from build123d import *

# Parameters (mm, degrees)
F1_DEPTH  = 16
F2_W      = 70
F2_H      = 3
F3_DEPTH  = 2
F4_W      = 50
F4_H      = 14
F5_DEPTH  = 2
F6_R      = 1
F9_DEPTH  = 2
F11_DEPTH = 38.001
F13_D     = 4
F14_R     = 2.999996841
F14_R_2   = 2
F15_DEPTH = 5
F16_R     = 3


# Not quite as in the source:
# - a pattern or mirror of a feature is missing from the dataset's text; its kind, count and spacing are read off the source's solid


with BuildPart() as f1:
    # F0 (on Front) → F1 (new body)
    with BuildSketch(Plane.XZ):
        with BuildLine():
            ThreePointArc((0, -9), (-9, 0), (0, 9))
            Line((0, 9), (94, 9))
            Line((94, 9), (94, 11))
            Line((94, 11), (0, 11))
            ThreePointArc((0, 11), (-11, 0), (0, -11))
            Line((0, -11), (19, -11))
            ThreePointArc((19, -11), (20.7464347921, -11.5607448848), (21.84, -13.0333563221))
            ThreePointArc((21.84, -13.0333563221), (39.3752187726, -41.0308955197), (67.5680682322, -58.2503420228))
            ThreePointArc((67.5680682322, -58.2503420228), (70.8216506695, -60.0087849904), (73.5012506711, -62.5578366136))
            Line((73.5012506711, -62.5578366136), (74.808430799, -61))
            ThreePointArc((74.808430799, -61), (71.3448519203, -57.9413219983), (67.1516242057, -56))
            ThreePointArc((67.1516242057, -56), (40.3930033582, -39.2216179023), (23.7333333333, -12.3889272035))
            ThreePointArc((23.7333333333, -12.3889272035), (21.9107246536, -9.9345748081), (19, -9))
            Line((19, -9), (0, -9))
        make_face()
    extrude(amount=F1_DEPTH)

    # F2 (on face) → F3 (join)
    with BuildSketch(Plane.XY.offset(11)):
        with Locations((59, -17.5)):
            Rectangle(F2_W, F2_H)
    extrude(amount=-F3_DEPTH)

    # F4 (on face) → F5 (join)
    with BuildSketch(Plane.XZ.offset(19)):
        with Locations((69, 2)):
            Rectangle(F4_W, F4_H)
    extrude(amount=-F5_DEPTH)

    # F6
    f6_edges = [f1.edges().sort_by_distance(p)[0] for p in [
        (59, -19, 11),
    ]]
    fillet(f6_edges, radius=F6_R)

    # F7: F1 across plane


with BuildPart() as f1_1:
    add(f1.part)
    add(f1.part.mirror(Plane.XZ))

    # F8 (on face) → F9 (cut)
    with BuildSketch(Plane.XY.offset(11)):
        with BuildLine():
            Line((33.7271293001, 11.9968971647), (34.2728706999, 11.9968971647))
            ThreePointArc((34.2728706999, 11.9968971647), (34, 12), (33.7271293001, 11.9968971647))
        make_face()
        with BuildLine():
            Line((94, 11.9968971647), (34.2728706999, 11.9968971647))
            Line((34.2728706999, 11.9968971647), (33.7271293001, 11.9968971647))
            ThreePointArc((33.7271293001, 11.9968971647), (22.0007757339, -0.1364441703), (34, -12))
            Line((34, -12), (94, -12))
            Line((94, -12), (94, 11.9968971647))
        make_face()
    extrude(amount=-F9_DEPTH, mode=Mode.SUBTRACT)

    # F10 (on face) → F11 (cut, through all)
    with BuildSketch(Plane.XZ.offset(19)):
        with BuildLine():
            ThreePointArc((50, 3), (47, 0), (50, -3))
            Line((50, -3), (70, -3))
            ThreePointArc((70, -3), (73, 0), (70, 3))
            Line((70, 3), (50, 3))
        make_face()
    extrude(amount=-F11_DEPTH, mode=Mode.SUBTRACT)

    # F13 (through all)
    with Locations(Plane.XZ.offset(19)):
        with Locations((80, 1)):
            Hole(F13_D / 2)

    # F14 (on face) → F15 (join)
    with BuildSketch(Plane(origin=(0, -17, 0), x_dir=(-1, 0, 0), z_dir=(0, 1, 0))):
        with Locations((-80, 1)):
            Circle(F14_R)
        with Locations((-80, 1)):
            Circle(F14_R_2, mode=Mode.SUBTRACT)
    f15 = extrude(amount=F15_DEPTH)

    # F15_copies: F15 across plane
    add(f15.mirror(Plane.ZX))

    # F16
    f16_edges = [f1_1.edges().sort_by_distance(p)[0] for p in [
        (94, -18, -5),
        (44, -18, -5),
        (94, 18, -5),
        (44, 18, -5),
    ]]
    fillet(f16_edges, radius=F16_R)


solid = f1_1.part
Input: part model. Units: mm. Frame: model coordinates. A direction names the side the tool comes from. Give positions to 0.01 mm unless a question says otherwise; leave off trailing zeros. Write each loop counter-clockwise with the first axis right and the second up, starting at its lowest first coordinate (ties: lowest second). Pieces come first, ordered by that corner, then holes.
Q1. Section C-C, the plane x = 86.5. Output: boundary loops of the cut face in (y, z), plus the area to 3 significant figures.
Q2. Section D-D, the plane z = 1. State how many separate pieces and enclosed holes the cut face has, plus the area to 3 significant figures.
Q3. Material intervals for probe 1 along Z at (x, y) = (80, -14); probe 2 along Z at (x, y) = (12.5, 8.5); probe 3 along Y at (x, z) = (75.5, 5), sorted ascending.
Q4. Set-up query: faces 1 (the face through (9, 0, -11)), 2 (the face through (77.14, -14.54, 1.9)), 3 (the face through (73, 18, 0)), 4 (the face through (22, 16, -12)). Return all of +Z, -Z, +X, -X, +Y, -Y with unobstructed straight access to the full face (end or side cutting, diameter ignored); none if empty.
Q5. First-contact query: P1, Ø1, axis at y = 9.5, z = 1.5, coming from the -X side; P2, Ø19, axis at x = 66, y = -7, coming from the -Z side; P3, Ø21, axis at x = 13, y = -3.5, coming from the -Z side. Flat tips, straight axial feed; report the tip coordinate or a pass-through.
Q6. Section A-A, the plane x = 16.5. Output: boundary loops of the cut face in (y, z).
Q7. Section B-B, the plane y = 0. Output: boundary loops of the cut face in (x, z), plus the area to 3 significant figures.
Q8. Pull-direction query (X, two-part tool) for faces 5 (the face through (78, -12, 0)), 6 (the face through (20.73, -0.22, -11.55)), 7 (the face through (47, -18, 0)); classes: pulls with the +X half, pulls with the -X half, needs draft (parallel to the pull), parting line crosses it, or undercut.
Filled in:
1. outline: (-19, -5) - (-17, -5) - (-17, 9) - (-12, 9) - (-12, 11) - (-18, 11) arc R1 ccw to (-19, 10) - close; (12, 9) - (17, 9) - (17, -5) - (19, -5) - (19, 10) arc R1 ccw to (18, 11) - (12, 11) - close
1. area: 83.6 mm2
2. separate pieces: 7
2. enclosed holes: 0
2. area: 166 mm2
3. probe 1: z = -2 to -1, 3 to 4, 9 to 11
3. probe 2: z = -11 to -9, 9 to 11
3. probe 3: y = -19 to -17, 17 to 19
4. face 1: -Z, -X, +Y, -Y
4. face 2: none
4. face 3: +Y, -Y
4. face 4: -Z, -X, +Y
5. P1: stops at x = -10.95
5. P2: stops at z = -62.56
5. P3: stops at z = -17.43
6. outline: (-16, -11) - (16, -11) - (16, -9) - (-16, -9) - close; (-16, 9) - (16, 9) - (16, 11) - (-16, 11) - close
7. outline: (0, -11) - (19, -11) arc R3 cw to (21.84, -13.03) arc R72 ccw to (67.57, -58.25) arc R14 cw to (73.5, -62.56) - (74.81, -61) arc R16 ccw to (67.15, -56) arc R70 cw to (23.73, -12.39) arc R5 ccw to (19, -9) - (0, -9) arc R9 cw to (0, 9) - (22, 9) - (22, 11) - (0, 11) arc R11 ccw to start
7. area: 302 mm2
8. face 5: needs draft
8. face 6: pulls with the -X half
8. face 7: undercut
